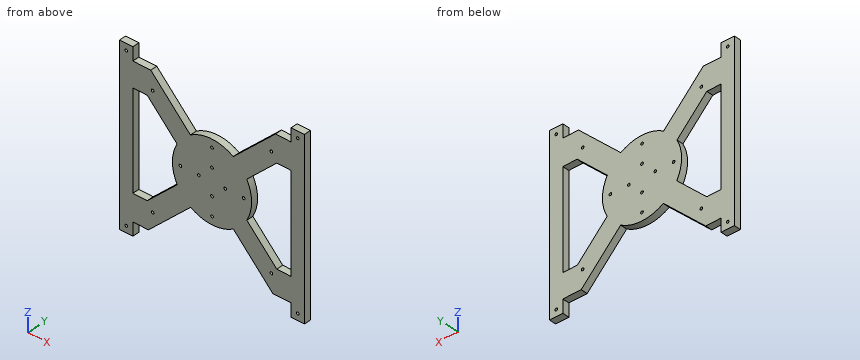
```python
from build123d import *

# Parameters (mm, degrees)
SKETCH1_R           = 1.27
BOSS_EXTRUDE1_DEPTH = 6.5278


with BuildPart() as part:
    # Sketch1 → Boss-Extrude1 (new body)
    with BuildSketch(Plane(origin=(0, 0, 0), x_dir=(1, 0, 0), z_dir=(0, 1, 0))):
        with BuildLine():
            Line((177.8, 0), (165.1, 0))
            Line((165.1, 0), (165.1, 12.7))
            Line((165.1, 12.7), (149.996873526, 12.7))
            Line((149.996873526, 12.7), (109.316778017, 51.969733907))
            ThreePointArc((109.316778017, 51.969733907), (88.681426877, 46.038126963), (68.115490096, 52.206102473))
            Line((68.115490096, 52.206102473), (29.979047387, 12.7))
            Line((29.979047387, 12.7), (12.7, 12.7))
            Line((12.7, 12.7), (12.7, 0))
            Line((12.7, 0), (0, 0))
            Line((0, 0), (0, 12.7))
            Line((0, 12.7), (0, 155.575))
            Line((0, 155.575), (0, 168.275))
            Line((0, 168.275), (12.7, 168.275))
            Line((12.7, 168.275), (12.7, 155.575))
            Line((12.7, 155.575), (27.681767073, 155.575))
            Line((27.681767073, 155.575), (68.410076297, 116.258723928))
            ThreePointArc((68.410076297, 116.258723928), (88.928296157, 122.237489492), (109.437612749, 116.228253537))
            Line((109.437612749, 116.228253537), (147.420224254, 155.575))
            Line((147.420224254, 155.575), (165.1, 155.575))
            Line((165.1, 155.575), (165.1, 168.275))
            Line((165.1, 168.275), (177.8, 168.275))
            Line((177.8, 168.275), (177.8, 155.575))
            Line((177.8, 155.575), (177.8, 12.7))
            Line((177.8, 12.7), (177.8, 0))
        make_face()
        with Locations((101.6, 84.1375)):
            Circle(SKETCH1_R, mode=Mode.SUBTRACT)
        with Locations((88.9, 71.4375)):
            Circle(SKETCH1_R, mode=Mode.SUBTRACT)
        with Locations((76.2, 84.1375)):
            Circle(SKETCH1_R, mode=Mode.SUBTRACT)
        with Locations((88.9, 96.8375)):
            Circle(SKETCH1_R, mode=Mode.SUBTRACT)
        with Locations((119.38, 84.1375)):
            Circle(SKETCH1_R, mode=Mode.SUBTRACT)
        with Locations((88.9, 53.6575)):
            Circle(SKETCH1_R, mode=Mode.SUBTRACT)
        with Locations((58.42, 84.1375)):
            Circle(SKETCH1_R, mode=Mode.SUBTRACT)
        with Locations((88.9, 114.6175)):
            Circle(SKETCH1_R, mode=Mode.SUBTRACT)
        with Locations((171.45, 161.925)):
            Circle(SKETCH1_R, mode=Mode.SUBTRACT)
        with Locations((171.45, 6.35)):
            Circle(SKETCH1_R, mode=Mode.SUBTRACT)
        with Locations((6.35, 6.35)):
            Circle(SKETCH1_R, mode=Mode.SUBTRACT)
        with Locations((6.35, 161.925)):
            Circle(SKETCH1_R, mode=Mode.SUBTRACT)
        with Locations((146.05, 138.225892857)):
            Circle(SKETCH1_R, mode=Mode.SUBTRACT)
        with Locations((146.05, 30.049107143)):
            Circle(SKETCH1_R, mode=Mode.SUBTRACT)
        with Locations((31.75, 30.049107143)):
            Circle(SKETCH1_R, mode=Mode.SUBTRACT)
        with Locations((31.75, 138.225892857)):
            Circle(SKETCH1_R, mode=Mode.SUBTRACT)
        with BuildLine():
            Line((165.1, 132.097774838), (165.1, 37.982848079))
            Line((165.1, 37.982848079), (151.23481924, 37.982848079))
            Line((151.23481924, 37.982848079), (122.338925223, 65.876933745))
            ThreePointArc((122.338925223, 65.876933745), (126.999904752, 84.052306631), (122.420253584, 102.248342047))
            Line((122.420253584, 102.248342047), (151.23481924, 132.097774838))
            Line((151.23481924, 132.097774838), (165.1, 132.097774838))
        make_face(mode=Mode.SUBTRACT)
        with BuildLine():
            Line((12.7, 130.175), (12.7, 36.592345569))
            Line((12.7, 36.592345569), (26.56518076, 36.592345569))
            Line((26.56518076, 36.592345569), (55.23682207, 66.293720925))
            ThreePointArc((55.23682207, 66.293720925), (50.800488469, 84.330427734), (55.41925789, 102.321281448))
            Line((55.41925789, 102.321281448), (26.56518076, 130.175))
            Line((26.56518076, 130.175), (12.7, 130.175))
        make_face(mode=Mode.SUBTRACT)
    extrude(amount=BOSS_EXTRUDE1_DEPTH)


solid = part.part
```
CAD build for the part. Positions are in the model's coordinates, mm. Round coordinates to 2 decimals unless told otherwise and drop trailing zeros. Loops run counter-clockwise (first coordinate to the right, second up) from the corner with the lowest first, then second, coordinate; pieces in that order, holes last. Notation, with made-up numbers: M -5.5,-34.5 L 10.5,-34.5 A26 ccw 10.5,-3.5 Z; hole C 26.5,-9.5 d11. An arc over 180 degrees is marked long. Use a Markdown table: item, result. Add a question column.
(1) Cut at C-C (x = 82). Give the cut face in (y, z), and give its area (3 significant figures).
(2) Flat gauge pins, fed straight in: pin 1 (1.5 mm diameter, centred on x = 96.5, y = 1.5, fed in from +Z); pin 2 (2 mm diameter, centred on x = 157.5, y = 3.5, fed in from +Z); pin 3 (3 mm diameter, centred on x = 103.5, y = 4, fed in from +Z). Where does each tip first touch, or does it go through?
(3) Drill centre lines: line 1 (Z direction, x = 88.9, y = 1.75); line 2 (Z direction, x = 31.75, y = 2.5); line 3 (X direction, y = 2.5, z = -6.35). Where is each one in solid material? Low to high.
(4) Cut at B-B (y = 3.5). State how many separate pieces and enclosed holes the cut face has, and give its area (3 significant figures).
(5) Cut at A-A (x = 130). Give the cut face in (y, z).
Geometry says:
| question | item | result |
|---|---|---|
| 1 | outline | M 0,-121.61 L 6.53,-121.61 L 6.53,-46.67 L 0,-46.67 Z |
| 1 | area | 489 mm² |
| 2 | pin 1 | stops at z = -46.66 |
| 2 | pin 2 | stops at z = -12.7 |
| 2 | pin 3 | stops at z = -48.36 |
| 3 | line 1 | z = -122.24 to -115.89, -113.35 to -98.11, -95.57 to -72.71, -70.17 to -54.93, -52.39 to -46.04 |
| 3 | line 2 | z = -151.65 to -139.5, -136.96 to -125.17, -41.96 to -31.32, -28.78 to -14.53 |
| 3 | line 3 | x = 0 to 5.08, 7.62 to 12.7, 165.1 to 170.18, 172.72 to 177.8 |
| 4 | separate pieces | 1 |
| 4 | enclosed holes | 18 |
| 4 | area | 13,800 mm² |
| 5 | outline | M 0,-137.53 L 6.53,-137.53 L 6.53,-110.1 L 0,-110.1 Z; M 0,-58.48 L 6.53,-58.48 L 6.53,-32 L 0,-32 Z |
